```python
from build123d import *

# Parameters (mm, degrees)
SKETCH1_W           = 260
SKETCH1_H           = 20
BOSS_EXTRUDE1_DEPTH = 5
SKETCH2_W           = 5
SKETCH2_H           = 20
BOSS_EXTRUDE2_DEPTH = 19
SKETCH3_R           = 2
CUT_EXTRUDE1_DEPTH  = 262.296766149
SKETCH4_W           = 5
SKETCH4_H           = 5
BOSS_EXTRUDE3_DEPTH = 5
CUT_EXTRUDE2_DEPTH  = 134.701159307
SKETCH6_R           = 2
CUT_EXTRUDE3_DEPTH  = 133.574507353


with BuildPart() as part:
    # Sketch1 → Boss-Extrude1 (new body)
    with BuildSketch(Plane.XY):
        Rectangle(SKETCH1_W, SKETCH1_H)
    extrude(amount=BOSS_EXTRUDE1_DEPTH)

    # Sketch2 → Boss-Extrude2 (add)
    with BuildSketch(Plane.XY.offset(5)):
        with Locations((127.5, 0)):
            Rectangle(SKETCH2_W, SKETCH2_H)
    extrude(amount=BOSS_EXTRUDE2_DEPTH)

    # Sketch3 → Cut-Extrude1 (cut, through all)
    with BuildSketch(Plane(origin=(130, 0, 0), x_dir=(0, 0, -1), z_dir=(1, 0, 0))):
        with Locations((-14.5, 0)):
            Circle(SKETCH3_R)
    extrude(amount=-CUT_EXTRUDE1_DEPTH, mode=Mode.SUBTRACT)

    # Sketch4 → Boss-Extrude3 (add)
    with BuildSketch(Plane.ZY.offset(-125)):
        with Locations((7.5, -7.5)):
            Rectangle(SKETCH4_W, SKETCH4_H)
        with Locations((7.5, 7.5)):
            Rectangle(SKETCH4_W, SKETCH4_H)
    extrude(amount=BOSS_EXTRUDE3_DEPTH)

    # Sketch5 → Cut-Extrude2 (cut, through all)
    with BuildSketch(Plane.XZ.offset(10)):
        Polygon((120, 5), (125, 10), (120, 10), align=None)
    extrude(amount=-CUT_EXTRUDE2_DEPTH, mode=Mode.SUBTRACT)

    # Sketch6 → Cut-Extrude3 (cut, through all)
    with BuildSketch(Plane(origin=(0, 0, 0), x_dir=(-1, 0, 0), z_dir=(0, 0, -1))):
        with Locations((118, 0)):
            Circle(SKETCH6_R)
    extrude(amount=-CUT_EXTRUDE3_DEPTH, mode=Mode.SUBTRACT)


solid = part.part
```
Can you work these out from the model? Positions are in its coordinate system, mm. A direction names the side the tool comes from. Coordinates: 2 decimals unless noted, no trailing zeros. Order: outer loops, then holes, each group sorted by start corner. A loop starts at its lowest first (then second) coordinate and runs counter-clockwise, first axis right, second up.
1. Thinking about a two-plate mould opening in X: for faces 3 (the face through (-1, 10, 3)), 4 (the face through (130, 0, 12)), 5 (the face through (-116, 0, 2)), 6 (the face through (-130, 0, 2)), which applies, +X half, -X half, draft (parallel to the pull), parting line (faces both ways), or undercut?
2. I'm going to push flat-ended pins straight in: pin 1 (6 mm diameter, centred on x = 20.5, y = -4.5, fed in from +Z); pin 2 (5.5 mm diameter, centred on y = -2, z = 13, fed in from -X); pin 3 (10 mm diameter, centred on x = 34, z = 9.5, fed in from -Y); pin 4 (2.5 mm diameter, centred on x = -118, y = 0, fed in from -Z). Where does each tip first touch, or does it pass through?
3. For faces 1 (the face through (123, -5, 7)), 2 (the face through (127, 0, 24)), which set-ups out of +Z, -Z, +X, -X, +Y, -Y let a thin tool reach every point of the face, with its end or its side?
4. I need wall thicknesses on line 1 (Y direction, x = 127, z = 14.5); line 2 (X direction, y = 3.75, z = 11.75); line 3 (Z direction, x = 56.5, y = 7.25). Which ranges of each line are inside material? Lowest first, please.
5. If we section it at B-B (z = 20.25): Please give me the cut outline in (x, y), then the cut area to 3 significant figures.
6. If we section it at A-A (x = 85): Please give me the cut outline in (y, z).
Entries:
1. face 3: draft
1. face 4: +X half
1. face 5: undercut
1. face 6: -X half
2. pin 1: stops at z = 5
2. pin 2: stops at x = 125
2. pin 3: stops at y = -10
2. pin 4: passes through
3. face 1: +Z, -X
3. face 2: +Z, +X, -X, +Y, -Y
4. line 1: y = -10 to -2, 2 to 10
4. line 2: x = 125 to 130
4. line 3: z = 0 to 5
5. outline: (125, -10) - (130, -10) - (130, 10) - (125, 10) - close
5. area: 100 mm2
6. outline: (-10, 0) - (10, 0) - (10, 5) - (-10, 5) - close
